```python
from build123d import *

# Parameters (mm, degrees)
SKETCH036_W     = 171
SKETCH036_H     = 171
PAD018_DEPTH    = 22
SKETCH037_W     = 167
SKETCH037_H     = 167
POCKET018_DEPTH = 21.5
SKETCH038_R     = 1.5
POCKET019_DEPTH = 171.001
SKETCH039_R     = 1.5
POCKET020_DEPTH = 171.001


with BuildPart() as part:
    # Sketch036 → Pad018 (new body)
    with BuildSketch(Plane.XY):
        with Locations((83, 83)):
            Rectangle(SKETCH036_W, SKETCH036_H)
    extrude(amount=PAD018_DEPTH)

    # Sketch037 (on Face5 of Pad018) → Pocket018 (cut)
    with BuildSketch(Plane(origin=(0, 0, 0), x_dir=(1, 0, 0), z_dir=(0, 0, -1))):
        with Locations((83, -83)):
            Rectangle(SKETCH037_W, SKETCH037_H)
    extrude(amount=-POCKET018_DEPTH, mode=Mode.SUBTRACT)

    # Sketch038 (on Face6 of Pocket018) → Pocket019 (cut, through all)
    with BuildSketch(Plane.XZ.offset(2.5)):
        with Locations((41.5, 3)):
            Circle(SKETCH038_R)
        with Locations((124.5, 3)):
            Circle(SKETCH038_R)
    extrude(amount=-POCKET019_DEPTH, mode=Mode.SUBTRACT)

    # Sketch039 (on Face5 of Pocket019) → Pocket020 (cut, through all)
    with BuildSketch(Plane.YZ.offset(168.5)):
        with Locations((47.981081, 3)):
            Circle(SKETCH039_R)
        with Locations((115.239796, 3)):
            Circle(SKETCH039_R)
    extrude(amount=-POCKET020_DEPTH, mode=Mode.SUBTRACT)


solid = part.part
```
Model file for the job. Use its own axes, mm. A direction names the side the tool comes from. Coordinates: 2 decimals unless noted, no trailing zeros. Order: outer loops, then holes, each group sorted by start corner. A loop starts at its lowest first (then second) coordinate and runs counter-clockwise, first axis right, second up. Notation, with made-up numbers: (-7, 33.25) - (17, 33.25) arc R27 ccw to (17, 64.25) - close; hole circle Ø1 at (75.25, 52.25). An arc over 180 degrees is marked (long way). Return JSON: item names as keys, results as strings. Group by question number.
1) Mould opens along X. For faces 3 (the flat face through (82, 168.5, 11)), 4 (the flat face through (166.5, 84, 11)), 5 (the flat face through (168.5, 82, 11)) say: released by +X, released by -X, zero draft, split by the parting line, or undercut.
2) Probe line 1 (X direction, y = 28.5, z = 15.75); line 2 (Z direction, x = 41.5, y = 167.7). List the from-to ranges inside material, lowest first. Write a range as from..to.
3) Tool access for faces 1 (the flat face through (-2.5, 82, 11)), 2 (the flat face through (82, 82, 21.5)): list every direction of +Z, -Z, +X, -X, +Y, -Y with a clear straight run to the whole face (end or side of a thin tool).
4) Flat gauge pins, fed straight in: P1, Ø2.5, axis at x = 124.5, z = 3, coming from the -Y side; P2, Ø1.5, axis at x = 99.5, y = 73, coming from the -Z side. Where does each tip first touch, or does it go through?
5) Saw through at B-B, the plane z = 16.5. Write the cut outline in (x, y), plus the area to 3 significant figures.
6) Saw through at A-A, the plane x = 52. Write the cut outline in (y, z).
Values found:
{
 "1": {"face 3": "zero draft", "face 4": "undercut", "face 5": "released by +X"},
 "2": {"line 1": "x = -2.5..-0.5, 166.5..168.5", "line 2": "z = 0..1.5, 4.5..22"},
 "3": {"face 1": "+Z, -Z, -X, +Y, -Y", "face 2": "-Z"},
 "4": {"P1": "passes through", "P2": "stops at z = 21.5"},
 "5": {"outline": "(-2.5, -2.5) - (168.5, -2.5) - (168.5, 168.5) - (-2.5, 168.5) - close; hole (-0.5, -0.5) - (166.5, -0.5) - (166.5, 166.5) - (-0.5, 166.5) - close", "area": "1,350 mm²"},
 "6": {"outline": "(-2.5, 0) - (-0.5, 0) - (-0.5, 21.5) - (166.5, 21.5) - (166.5, 0) - (168.5, 0) - (168.5, 22) - (-2.5, 22) - close"}
}
